Check sheet for the modelled part. Datum: model origin and axes. Units: mm. A direction names the side the tool comes from. Coordinates: 2 decimals unless noted, no trailing zeros. Loops run counter-clockwise (first coordinate to the right, second up) from the corner with the lowest first, then second, coordinate; pieces in that order, holes last. Notation, with made-up numbers: (74, 68) - (110, 68) arc R25 cw to (110, 93) - close; hole circle Ø7 at (11, 48). An arc over 180 degrees is marked (long way). Use a Markdown table: item, result. Add a question column.
1) Sectioned sample at A-A, the plane z = -4.25. Enter the section's corners in (x, y).
2) Sectioned sample at C-C, the plane z = 8. Enter the section's corners in (x, y), then the cut area to 3 significant figures.
3) Draft check along X on faces 4 (the flat face through (0, -21.998, 11)), 5 (the conical face through (-0.036, -42.669, 0.707)), 6 (the flat face through (4.5, -13, 11)). Enter one of: pulls with the +X half, pulls with the -X half, needs draft (parallel to the pull), parting line crosses it, or undercut.
4) Sectioned sample at B-B, the plane y = -32.5. Enter the section's corners in (x, z).
5) Thickness scan on line 1 (Y direction, x = 0, z = -4.5); line 2 (X direction, y = -49, z = 0.25); line 3 (Y direction, x = 3.7, z = 3). Record the ranges inside material, lowest first.
6) Tool access check on faces 1 (the flat face through (-4.4, -39.7, 6.5)), 2 (the flat face through (0, -22.498, 8)), 3 (the cylindrical face through (-0.16, -34.96, -3.2)). Record the directions out of +Z, -Z, +X, -X, +Y, -Y that give a thin tool (end or side, any length) a straight path to the whole face; none if there is none.
7) Go/stop test with flat-tipped pins: P1, Ø0.8, axis at x = -4.5, z = 6.5, coming from the +Y side; P2, Ø0.8, axis at y = -16, z = 11, coming from the -X side; P3, Ø2.5, axis at x = 2, z = 8.5, coming from the -Y side; P4, Ø5, axis at x = -1, y = -27.5, coming from the +Z side. Record where each tip stops, or that it passes through.
from build123d import *

# Parameters (mm, degrees)
SKETCH1_W                         = 10
SKETCH1_H                         = 14
EXTRUDE1_DEPTH                    = 56.7
SKETCH2_W                         = 10
SKETCH2_H                         = 18.498
EXTRUDE2_DEPTH                    = 3
M3X0_5_TAPPED_HOLE1_D             = 2.5
M3X0_5_TAPPED_HOLE1_DEPTH         = 7.5
M3X0_5_TAPPED_HOLE1_TIP           = 0.220408726
SKETCH5_R                         = 1.05
MANIFOLD_SCREWS_COUNTERBORE_DEPTH = 15
SKETCH6_R                         = 1.05
MOUNTING_HOLE_DEPTH               = 1
SKETCH7_W                         = 9
SKETCH7_H                         = 17.498
EXTRUDE3_DEPTH                    = 3.5
FILLET1_R                         = 1


with BuildPart() as part:
    # Sketch1 → Extrude1 (new body)
    with BuildSketch(Plane(origin=(0, 0, 0), x_dir=(1, 0, 0), z_dir=(0, 1, 0))):
        Rectangle(SKETCH1_W, SKETCH1_H)
    extrude(amount=-EXTRUDE1_DEPTH)

    # Sketch2 → Extrude2 (add)
    with BuildSketch(Plane.XY.offset(7)):
        with Locations((0, -13.249)):
            Rectangle(SKETCH2_W, SKETCH2_H)
    extrude(amount=EXTRUDE2_DEPTH)

    # M3x0.5 Tapped Hole1
    with Locations(Plane(origin=(0, -36.2, -7), x_dir=(-1, 0, 0), z_dir=(0, 0, -1))):
        with Locations((0, 0), (0, -6.4), (0, -12.8), (2, -9.6), (-2, -3.2)):
            Hole(M3X0_5_TAPPED_HOLE1_D / 2, depth=M3X0_5_TAPPED_HOLE1_DEPTH)
            with Locations((0, 0, -(M3X0_5_TAPPED_HOLE1_DEPTH + M3X0_5_TAPPED_HOLE1_TIP / 2))):  # 160° drill point
                Cone(0, M3X0_5_TAPPED_HOLE1_D / 2, M3X0_5_TAPPED_HOLE1_TIP, mode=Mode.SUBTRACT)

    # Sketch5 → Manifold Screws Counterbore (cut, through all)
    with BuildSketch(Plane.XY.offset(7)):
        with Locations((-3.7, -38.1)):
            Circle(SKETCH5_R)
        with Locations((3.7, -47.4)):
            Circle(SKETCH5_R)
    extrude(amount=-MANIFOLD_SCREWS_COUNTERBORE_DEPTH, mode=Mode.SUBTRACT)

    # Sketch6 → Mounting Hole (cut)
    with BuildSketch(Plane.XY.offset(7)):
        with BuildLine():
            ThreePointArc((-2.1, -38.1), (-2.56862915, -36.96862915), (-3.7, -36.5))
            ThreePointArc((-3.7, -36.5), (-4.4306228, -36.676556877), (-5, -37.167262095))
            Line((-5, -37.167262095), (-5, -39.032737905))
            ThreePointArc((-5, -39.032737905), (-4.4306228, -39.523443123), (-3.7, -39.7))
            ThreePointArc((-3.7, -39.7), (-2.56862915, -39.23137085), (-2.1, -38.1))
        make_face()
        with Locations((-3.7, -38.1)):
            Circle(SKETCH6_R, mode=Mode.SUBTRACT)
        with BuildLine():
            Line((5, -48.332737905), (5, -46.467262095))
            ThreePointArc((5, -46.467262095), (4.4306228, -45.976556877), (3.7, -45.8))
            ThreePointArc((3.7, -45.8), (2.1, -47.4), (3.7, -49))
            ThreePointArc((3.7, -49), (4.4306228, -48.823443123), (5, -48.332737905))
        make_face()
        with Locations((3.7, -47.4)):
            Circle(SKETCH6_R, mode=Mode.SUBTRACT)
        with BuildLine():
            Line((5, -46.467262095), (5, -45.8))
            Line((5, -45.8), (3.7, -45.8))
            ThreePointArc((3.7, -45.8), (4.4306228, -45.976556877), (5, -46.467262095))
        make_face()
        with BuildLine():
            Line((5, -49), (5, -48.332737905))
            ThreePointArc((5, -48.332737905), (4.4306228, -48.823443123), (3.7, -49))
            Line((3.7, -49), (5, -49))
        make_face()
        with BuildLine():
            ThreePointArc((-5, -37.167262095), (-4.4306228, -36.676556877), (-3.7, -36.5))
            Line((-3.7, -36.5), (-5, -36.5))
            Line((-5, -36.5), (-5, -37.167262095))
        make_face()
        with BuildLine():
            Line((-5, -39.7), (-3.7, -39.7))
            ThreePointArc((-3.7, -39.7), (-4.4306228, -39.523443123), (-5, -39.032737905))
            Line((-5, -39.032737905), (-5, -39.7))
        make_face()
    extrude(amount=-MOUNTING_HOLE_DEPTH, mode=Mode.SUBTRACT)

    # Sketch7 → Extrude3 (add)
    with BuildSketch(Plane.XY.offset(10)):
        with Locations((0, -13.249)):
            Rectangle(SKETCH7_W, SKETCH7_H)
    extrude(amount=EXTRUDE3_DEPTH)

    # Fillet1
    fillet1_edges = [part.edges().sort_by_distance(p)[0] for p in [
        (0, -4.5, 13.5),
        (-4.5, -13.249, 13.5),
        (0, -21.998, 13.5),
        (4.5, -13.249, 13.5),
    ]]
    fillet(fillet1_edges, radius=FILLET1_R)


solid = part.part
Solved:
| question | item | result |
|---|---|---|
| 1 | outline | (-5, -56.7) - (5, -56.7) - (5, 0) - (-5, 0) - close; hole circle Ø2.1 at (-3.7, -38.1); hole circle Ø2.5 at (-2, -45.8); hole circle Ø2.5 at (0, -49); hole circle Ø2.5 at (0, -42.6); hole circle Ø2.5 at (0, -36.2); hole circle Ø2.5 at (2, -39.4); hole circle Ø2.1 at (3.7, -47.4) |
| 2 | outline | (-5, -22.5) - (5, -22.5) - (5, -4) - (-5, -4) - close |
| 2 | area | 185 mm2 |
| 3 | face 4 | needs draft |
| 3 | face 5 | undercut |
| 3 | face 6 | pulls with the +X half |
| 4 | outline | (-5, -7) - (5, -7) - (5, 7) - (-5, 7) - close |
| 5 | line 1 | y = -56.7 to -50.25, -47.75 to -43.85, -41.35 to -37.45, -34.95 to 0 |
| 5 | line 2 | x = -5 to -1.25, 1.25 to 5 |
| 5 | line 3 | y = -56.7 to -48.45, -46.35 to 0 |
| 6 | face 1 | +Z, -X |
| 6 | face 2 | +Z, +X, -X, -Y |
| 6 | face 3 | -Z |
| 7 | P1 | stops at y = 0 |
| 7 | P2 | stops at x = -4.5 |
| 7 | P3 | stops at y = -22.5 |
| 7 | P4 | stops at z = 7 |
